Check sheet for the drawn part. Datum: minimum x, y, z corner. Units: mm. A direction names the side the tool comes from. Give positions to 0.01 mm unless a question says otherwise; leave off trailing zeros. Order: outer loops, then holes, each group sorted by start corner. A loop starts at its lowest first (then second) coordinate and runs counter-clockwise, first axis right, second up.
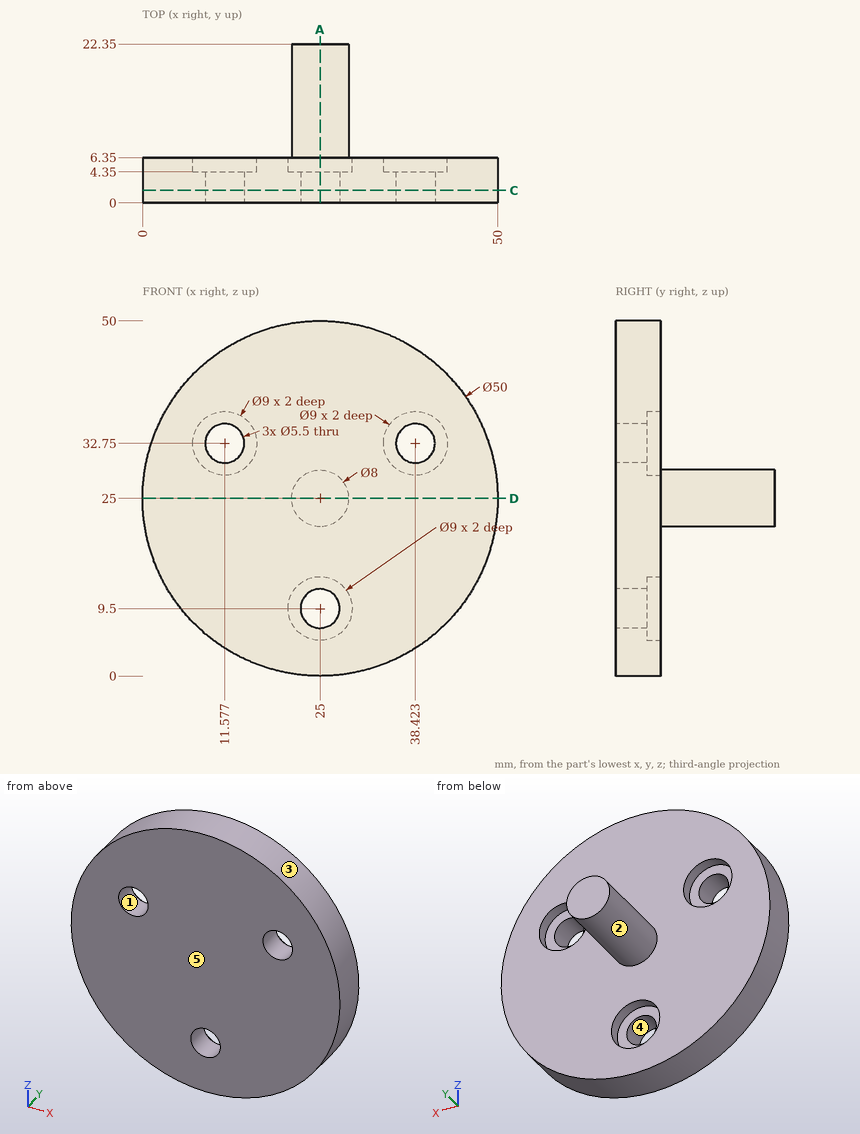
(1) Section check C-C, the plane y = 1.75. Enter the section's corners in (x, z), then the cut area to 3 significant figures.
Solved:
outline: circle Ø50 at (25, 25); hole circle Ø5.5 at (11.58, 32.75); hole circle Ø5.5 at (25, 9.5); hole circle Ø5.5 at (38.42, 32.75)
area: 1,890 mm2
(2) Section check D-D, the plane z = 25. Enter the section's corners in (x, y).
Solved:
outline: (0, 0) - (50, 0) - (50, 6.35) - (29, 6.35) - (29, 22.35) - (21, 22.35) - (21, 6.35) - (0, 6.35) - close
(3) Set-up check for the marked faces 1 and 2: record each of +Z, -Z, +X, -X, +Y, -Y from which the full face is reachable in a straight line by a thin tool's end or side.
Solved:
face 1: +Y, -Y
face 2: +Y
(4) Section check A-A, the plane x = 25. Enter the section's corners in (y, z).
Solved:
outline: (0, 0) - (6.35, 0) - (6.35, 5) - (4.35, 5) - (4.35, 6.75) - (0, 6.75) - close; (0, 12.25) - (4.35, 12.25) - (4.35, 14) - (6.35, 14) - (6.35, 21) - (22.35, 21) - (22.35, 29) - (6.35, 29) - (6.35, 50) - (0, 50) - close
(5) Release check for a two-part mould opening along X. For the marked faces 3, 4 and 5 record: pulls with the +X half, pulls with the -X half, needs draft (parallel to the pull), parting line crosses it, or undercut.
Solved:
face 3: parting line crosses it
face 4: undercut
face 5: needs draft
(6) Scan lines: line 1 (Y direction, x = 9, z = 36); line 2 (Y direction, x = 15, z = 22); line 3 (X direction, y = 18, z = 28.5) (1 decimal). Record each from-to range of solid material in increasing order.
Solved:
line 1: y = 0 to 4.35
line 2: y = 0 to 6.35
line 3: x = 23.1 to 26.9
(7) Go/stop test with flat-tipped pins: pin 1 (10 mm diameter, centred on x = 38, z = 32, fed in from +Y); pin 2 (8 mm diameter, centred on x = 26.5, y = 13, fed in from +Z); pin 3 (8 mm diameter, centred on y = 10, z = 24, fed in from -X). Record where each tip stops, or that it passes through.
Solved:
pin 1: stops at y = 6.35
pin 2: stops at z = 29
pin 3: stops at x = 0
